```python
from build123d import *

# Parameters (mm, degrees)
SKETCH1_W           = 162.56
SKETCH1_H           = 73.66
BOSS_EXTRUDE1_DEPTH = 5.08
SKETCH2_W           = 54.186666666
SKETCH2_H           = 5.08
CUT_EXTRUDE1_DEPTH  = 90.379492614
SKETCH5_W           = 2.7559
SKETCH5_H           = 13.081
CUT_EXTRUDE4_DEPTH  = 90.379492614
SKETCH6_W           = 6.096
SKETCH6_H           = 2.1717
CUT_EXTRUDE5_DEPTH  = 90.379492614
CAVITY1_START       = -36.83
CAVITY1_OUTLINE_W   = 5.08
CAVITY1_OUTLINE_H   = 5.08
CAVITY1_DEPTH       = 24.553333333
CAVITY1_START_2     = 12.276666667
CAVITY1_2_OUTLINE_W = 5.08
CAVITY1_2_OUTLINE_H = 5.08
CAVITY1_2_DEPTH     = 24.553333333


# Read off the part's stored shape, not the designer's step: Cavity1
with BuildPart() as part:
    # Sketch1 → Boss-Extrude1 (new body)
    with BuildSketch(Plane.XY):
        Rectangle(SKETCH1_W, SKETCH1_H)
    extrude(amount=BOSS_EXTRUDE1_DEPTH)

    # Sketch2 → Cut-Extrude1 (cut, through all)
    with BuildSketch(Plane.XY.offset(5.08)):
        with Locations((0, -34.29)):
            Rectangle(SKETCH2_W, SKETCH2_H)
        with Locations((0, 34.29)):
            Rectangle(SKETCH2_W, SKETCH2_H)
    extrude(amount=-CUT_EXTRUDE1_DEPTH, mode=Mode.SUBTRACT)

    # Sketch5 → Cut-Extrude4 (cut, through all)
    with BuildSketch(Plane.XY.offset(5.08)):
        with Locations((0, 25.2095)):
            Rectangle(SKETCH5_W, SKETCH5_H)
    extrude(amount=-CUT_EXTRUDE4_DEPTH, mode=Mode.SUBTRACT)

    # Sketch6 → Cut-Extrude5 (cut, through all)
    with BuildSketch(Plane.XY.offset(5.08)):
        with Locations((0, 25.2095)):
            Rectangle(SKETCH6_W, SKETCH6_H)
    extrude(amount=-CUT_EXTRUDE5_DEPTH, mode=Mode.SUBTRACT)

    # Cavity1 outline → Cavity1 (cut)
    with BuildSketch(Plane(origin=(0, 0, 0), x_dir=(1, 0, 0), z_dir=(0, 1, 0)).offset(CAVITY1_START)):
        with Locations((78.74, -2.54)):
            Rectangle(CAVITY1_OUTLINE_W, CAVITY1_OUTLINE_H)
        with Locations((-78.74, -2.54)):
            Rectangle(CAVITY1_OUTLINE_W, CAVITY1_OUTLINE_H)
    extrude(amount=CAVITY1_DEPTH, mode=Mode.SUBTRACT)

    # Cavity1 2 outline → Cavity1 2 (cut)
    with BuildSketch(Plane(origin=(0, 0, 0), x_dir=(1, 0, 0), z_dir=(0, 1, 0)).offset(CAVITY1_START_2)):
        with Locations((78.74, -2.54)):
            Rectangle(CAVITY1_2_OUTLINE_W, CAVITY1_2_OUTLINE_H)
        with Locations((-78.74, -2.54)):
            Rectangle(CAVITY1_2_OUTLINE_W, CAVITY1_2_OUTLINE_H)
    extrude(amount=CAVITY1_2_DEPTH, mode=Mode.SUBTRACT)


solid = part.part
```
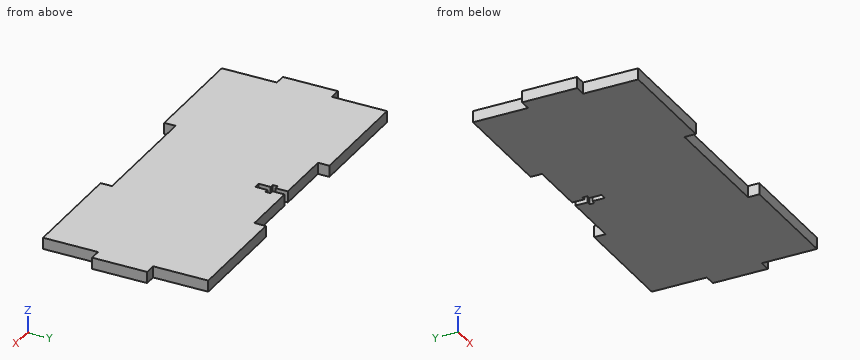
Here's how the part is built. I have some questions about the finished solid (model axes, mm). Coordinates: 2 decimals unless noted, no trailing zeros. Loops run counter-clockwise (first coordinate to the right, second up) from the corner with the lowest first, then second, coordinate; pieces in that order, holes last. Notation, with made-up numbers: (-5, 32) - (36, 32) arc R20 cw to (36, 43) - close; hole circle Ø10 at (8.25, -32). An arc over 180 degrees is marked (long way). Return JSON: item names as keys, results as strings. Group by question number.
Item 1: If we section it at C-C on x = -9: Write out the boundary of the cut face in (y, z), and give its area (3 significant figures).
Item 2: Will these pins go through, and if not, where does the flat tip stop? P1, Ø1.5, axis at y = 33.5, z = 2, coming from the +X side; P2, Ø0.8, axis at x = 0, z = 3.5, coming from the +Y side; P3, Ø1.5, axis at y = 26.5, z = 2.5, coming from the -X side.
Item 3: I need wall thicknesses on line 1 (X direction, y = 20, z = 1.6); line 2 (Y direction, x = 0.5, z = 1.65); line 3 (X direction, y = 16, z = 1.95). Which ranges of each line are inside material? Lowest first, please. Write a range as from..to.
Item 4: If we section it at B-B on y = -29.5: Write out the boundary of the cut face in (x, z), and give its area (3 significant figures).
Calculated:
{
 "1": {"outline": "(-31.75, 0) - (31.75, 0) - (31.75, 5.08) - (-31.75, 5.08) - close", "area": "323 mm^2"},
 "2": {"P1": "stops at x = 76.2", "P2": "stops at y = 18.67", "P3": "stops at x = -76.2"},
 "3": {"line 1": "x = -76.2..-1.38, 1.38..76.2", "line 2": "y = -31.75..18.67", "line 3": "x = -76.2..76.2"},
 "4": {"outline": "(-76.2, 0) - (76.2, 0) - (76.2, 5.08) - (-76.2, 5.08) - close", "area": "774 mm^2"}
}
